Source: CAD feature listing. Evaluate the final solid. Frame: model axes, mm. Coordinates: 2 decimals unless noted, no trailing zeros. Loops run counter-clockwise (first coordinate to the right, second up) from the corner with the lowest first, then second, coordinate; pieces in that order, holes last.
```python
from build123d import *

# Parameters (mm, degrees)
SKETCH1_R           = 2.75
BOSS_EXTRUDE1_DEPTH = 4
CUT_EXTRUDE1_DEPTH  = 10
BOSS_EXTRUDE3_START = -4
SKETCH3_R           = 2.75
BOSS_EXTRUDE3_DEPTH = 4
BOSS_EXTRUDE4_START = -4
SKETCH4_R           = 2.75
BOSS_EXTRUDE4_DEPTH = 4


with BuildPart() as part:
    # Sketch1 → Boss-Extrude1 (new body)
    with BuildSketch(Plane.XY):
        with BuildLine():
            Line((24.072178339, 16.5927117), (-24.072178339, 16.5927117))
            ThreePointArc((-24.072178339, 16.5927117), (-24.779285121, 16.299818481), (-25.072178339, 15.5927117))
            Line((-25.072178339, 15.5927117), (-25.072178339, 8.49545414))
            ThreePointArc((-25.072178339, 8.49545414), (-24.955491664, 8.026671065), (-24.632663198, 7.667289468))
            Line((-24.632663198, 7.667289468), (-1.120969717, -8.244942286))
            ThreePointArc((-1.120969717, -8.244942286), (0, -8.588612943), (1.120969717, -8.244942286))
            Line((1.120969717, -8.244942286), (24.632663198, 7.667289468))
            ThreePointArc((24.632663198, 7.667289468), (24.955491664, 8.026671065), (25.072178339, 8.49545414))
            Line((25.072178339, 8.49545414), (25.072178339, 15.5927117))
            ThreePointArc((25.072178339, 15.5927117), (24.779285121, 16.299818481), (24.072178339, 16.5927117))
        make_face()
        Circle(SKETCH1_R, mode=Mode.SUBTRACT)
        with Locations((-16.827094957, 10.809665828)):
            Circle(SKETCH1_R, mode=Mode.SUBTRACT)
        with Locations((16.827094957, 10.809665828)):
            Circle(SKETCH1_R, mode=Mode.SUBTRACT)
    extrude(amount=BOSS_EXTRUDE1_DEPTH)

    # Sketch2 → Cut-Extrude1 (cut)
    with BuildSketch(Plane.XY.offset(4)):
        Polygon((-24.632663198, 7.667289468), (24.632663198, 7.667289468), (0.25604332, -10.053182783), align=None)
    extrude(amount=-CUT_EXTRUDE1_DEPTH, mode=Mode.SUBTRACT)

    # Sketch3 → Boss-Extrude3 (add)
    # profile 1 of 2: a face of its own
    with BuildSketch(Plane.XY.offset(4).offset(BOSS_EXTRUDE3_START)):
        with BuildLine():
            Line((-24.072178339, 16.5927117), (-25.072178339, 16.5927117))
            Line((-25.072178339, 16.5927117), (-25.072178339, 15.5927117))
            ThreePointArc((-25.072178339, 15.5927117), (-24.779285121, 16.299818481), (-24.072178339, 16.5927117))
        make_face()
    # profile 2 of 2: a face of its own
    with BuildSketch(Plane.XY.offset(4).offset(BOSS_EXTRUDE3_START)):
        with BuildLine():
            ThreePointArc((-24.632663198, 7.667289468), (-24.955491664, 8.026671065), (-25.072178339, 8.49545414))
            Line((-25.072178339, 8.49545414), (-25.072178339, 2.887491698))
            Line((-25.072178339, 2.887491698), (75.267657001, 2.887491698))
            Line((75.267657001, 2.887491698), (75.267657001, 16.5927117))
            Line((75.267657001, 16.5927117), (24.072178339, 16.5927117))
            ThreePointArc((24.072178339, 16.5927117), (24.779285121, 16.299818481), (25.072178339, 15.5927117))
            Line((25.072178339, 15.5927117), (25.072178339, 8.49545414))
            ThreePointArc((25.072178339, 8.49545414), (24.955491664, 8.026671065), (24.632663198, 7.667289468))
            Line((24.632663198, 7.667289468), (-24.632663198, 7.667289468))
        make_face()
        with Locations((67.022573618, 10.809665828)):
            Circle(SKETCH3_R, mode=Mode.SUBTRACT)
    extrude(amount=BOSS_EXTRUDE3_DEPTH)

    # Sketch4 → Boss-Extrude4 (add)
    with BuildSketch(Plane.XY.offset(4).offset(BOSS_EXTRUDE4_START)):
        with Locations((16.827094957, 10.809665828)):
            Circle(SKETCH4_R)
    extrude(amount=BOSS_EXTRUDE4_DEPTH)


solid = part.part
```
Q1. Material intervals for line 1 along X through (y, z) = (9.75, 2.9); line 2 along X through (y, z) = (12, 1.45); line 3 along Y through (x, z) = (-15.5, 0.6), sorted ascending.
Q2. Draft query along Y for faces 1 (the flat face through (26, 16.593, 2)), 2 (the flat face through (-25.072, 10, 2)), 3 (the cylindrical face through (64.275, 10.931, 1.972)). Return one class per face: released by +Y, released by -Y, zero draft, split by the parting line, or undercut.
Q3. Section query A-A on y = 12. Return the cut outline in (x, z).
Q4. First-contact query: pin 1 Ø3.5 at (x, y) = (-16.83, 10.81) entering from -Z; pin 2 Ø6.5 at (x, y) = (67.02, 10.81) entering from -Z. Flat tips, straight axial feed; report the tip coordinate or a pass-through.
Q5. Section query B-B on z = 1. Return the cut outline in (x, y), then the cut area to 3 significant figures.
Resolved:
1. line 1: x = -25.07 to -19.36, -14.29 to 64.48, 69.56 to 75.27
1. line 2: x = -25.07 to -19.31, -14.35 to 64.54, 69.5 to 75.27
1. line 3: y = 2.89 to 8.4, 13.22 to 16.59
2. face 1: released by +Y
2. face 2: zero draft
2. face 3: undercut
3. outline: (-25.07, 0) - (-19.31, 0) - (-19.31, 4) - (-25.07, 4) - close; (-14.35, 0) - (64.54, 0) - (64.54, 4) - (-14.35, 4) - close; (69.5, 0) - (75.27, 0) - (75.27, 4) - (69.5, 4) - close
4. pin 1: passes through
4. pin 2: stops at z = 0
5. outline: (-25.07, 2.89) - (75.27, 2.89) - (75.27, 16.59) - (-25.07, 16.59) - close; hole circle Ø5.5 at (-16.83, 10.81); hole circle Ø5.5 at (67.02, 10.81)
5. area: 1,330 mm2
